from build123d import *

# Parameters (mm, degrees)
SKETCH010_W     = 220
SKETCH010_H     = 102
SKETCH010_W_2   = 150
SKETCH010_H_2   = 6
PAD006_DEPTH    = 10
SKETCH012_W     = 30
SKETCH012_H     = 102
SKETCH012_W_2   = 50
PAD007_DEPTH    = 19.5
CHAMFER001_SIZE = 1
SKETCH_R        = 2.55
HOLE_DEPTH      = 29.501


with BuildPart() as part:
    # Sketch010 → Pad006 (new body)
    with BuildSketch(Plane.XY):
        with BuildLine():
            Line((-150, 71), (-150, -71))
            ThreePointArc((-150, -71), (-148.828427, -73.828427), (-146, -75))
            Line((-146, -75), (146, -75))
            ThreePointArc((146, -75), (148.828427, -73.828427), (150, -71))
            Line((150, -71), (150, 71))
            ThreePointArc((150, 71), (148.828427, 73.828427), (146, 75))
            Line((146, 75), (-146, 75))
            ThreePointArc((-146, 75), (-148.828427, 73.828427), (-150, 71))
        make_face()
        with Locations((10, 0)):
            Rectangle(SKETCH010_W, SKETCH010_H, mode=Mode.SUBTRACT)
        with Locations((-25, 63)):
            Rectangle(SKETCH010_W_2, SKETCH010_H_2, mode=Mode.SUBTRACT)
        with Locations((-25, -63)):
            Rectangle(SKETCH010_W_2, SKETCH010_H_2, mode=Mode.SUBTRACT)
    extrude(amount=PAD006_DEPTH)

    # Sketch012 (on Face21 of Pad006) → Pad007 (join)
    with BuildSketch(Plane(origin=(0, 0, 0), x_dir=(1, 0, 0), z_dir=(0, 0, -1))):
        with Locations((135, 0)):
            Rectangle(SKETCH012_W, SKETCH012_H)
        with Locations((-125, 0)):
            Rectangle(SKETCH012_W_2, SKETCH012_H)
    extrude(amount=PAD007_DEPTH)

    # Chamfer001
    chamfer001_edges = [part.edges().sort_by_distance(p)[0] for p in [
        (-25, -66, 0),
        (-100, -63, 0),
        (-25, -60, 0),
        (50, -63, 0),
        (50, 63, 0),
        (-25, 66, 0),
        (-25, 60, 0),
        (-100, 63, 0),
        (-150, 0, -19.5),
        (-125, 51, -19.5),
        (-100, 0, -19.5),
        (-125, -51, -19.5),
        (120, 0, -19.5),
        (135, 51, -19.5),
        (150, 0, -19.5),
        (135, -51, -19.5),
        (0, -75, 0),
        (0, 75, 0),
        (10, -51, 0),
        (10, 51, 0),
        (-150, 0, 10),
        (-148.828427, -73.828427, 10),
        (0, -75, 10),
        (148.828427, -73.828427, 10),
        (150, 0, 10),
        (148.828427, 73.828427, 10),
        (0, 75, 10),
        (-148.828427, 73.828427, 10),
        (-100, 0, 10),
        (10, -51, 10),
        (120, 0, 10),
        (10, 51, 10),
        (-100, -63, 10),
        (-25, -66, 10),
        (50, -63, 10),
        (-25, -60, 10),
        (-100, 63, 10),
        (-25, 60, 10),
        (50, 63, 10),
        (-25, 66, 10),
    ]]
    chamfer(chamfer001_edges, length=CHAMFER001_SIZE)

    # Sketch (on Face15 of Chamfer001) → Hole (cut, through all)
    with BuildSketch(Plane.XY.offset(10)):
        with Locations((-130, 0)):
            Circle(SKETCH_R)
    extrude(amount=-HOLE_DEPTH, mode=Mode.SUBTRACT)


solid = part.part
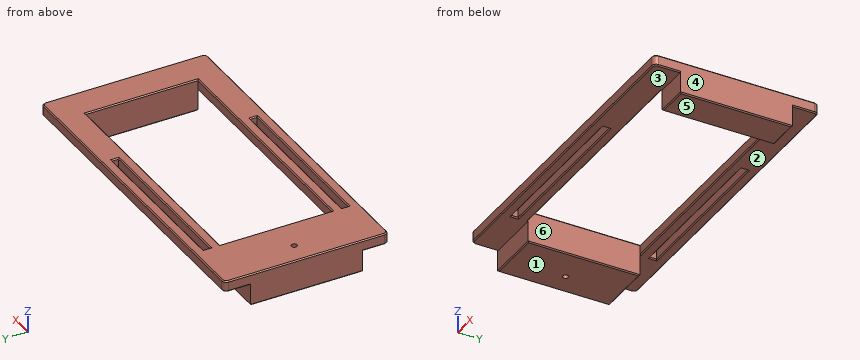
Design review of the part built by this model. Coordinates are the model's own, in mm. Face numbers are marked on the shaded views. A direction names the side the tool comes from. Round coordinates to 2 decimals unless told otherwise and drop trailing zeros. Write each loop counter-clockwise with the first axis right and the second up, starting at its lowest first coordinate (ties: lowest second). Pieces come first, ordered by that corner, then holes. Notation, with made-up numbers: (69, -20) - (91, -20) arc R17 cw to (91, -16) - close; hole circle Ø9 at (63, -20). An arc over 180 degrees is marked (long way). Return JSON: item names as keys, results as strings. Group by question number.
Item 1: Machinability: for the marked faces 1, 2 and 3, which of the approach directions +Z, -Z, +X, -X, +Y, -Y give a long, thin tool a straight path to every point of the face, cutting with its end or side? Answer none if there is none.
Item 2: We need section A-A on y = 31.5. Write out the cut boundary in (x, z).
Item 3: Insertion check: P1, Ø10, axis at x = 113.5, y = -24, coming from the -Z side; P2, Ø3, axis at x = 106, z = 0, coming from the +Y side; P3, Ø15.5, axis at x = -120.5, z = -10, coming from the -Y side; P4, Ø7, axis at x = -50, y = 58.5, coming from the -Z side. Each pin has a flat end and moves straight along its axis. Give the tip position at first contact, or say it passes through.
Item 4: The part is to be moulded in two halves that separate along X. For the marked faces 4, 5 and 6, say which applies: pulls with the +X half, pulls with the -X half, needs draft (parallel to the pull), parting line crosses it, or undercut.
Item 5: We need section B-B on z = -6.5. Write out the cut boundary in (x, y), and give its area (3 significant figures).
Item 6: For probe 1 along Y at (x, z) = (-13.5, 7.75); probe 2 along X at (y, z) = (-24.5, 0); probe 3 along Y at (x, z) = (-130, -4), list the stretches that pass through material, from the lowest coordinate up. Write a range as [from, to].
Item 7: We need section C-C on x = 101. Write out the cut boundary in (y, z).
Model answer:
{
 "1": {"face 1": "-Z, +X, -X, +Y, -Y", "face 2": "-Z, +X, -X, +Y", "face 3": "-Z, +X, -X, -Y"},
 "2": {"outline": "(-150, -18.5) - (-149, -19.5) - (-101, -19.5) - (-100, -18.5) - (-100, 9) - (-101, 10) - (-149, 10) - (-150, 9) - close; (120, -18.5) - (121, -19.5) - (149, -19.5) - (150, -18.5) - (150, 9) - (149, 10) - (121, 10) - (120, 9) - close"},
 "3": {"P1": "passes through", "P2": "stops at y = 75", "P3": "stops at y = -51", "P4": "stops at z = 0"},
 "4": {"face 4": "pulls with the +X half", "face 5": "needs draft", "face 6": "undercut"},
 "5": {"outline": "(-150, -51) - (-100, -51) - (-100, 51) - (-150, 51) - close; (120, -51) - (150, -51) - (150, 51) - (120, 51) - close; hole circle Ø5.1 at (-130, 0)", "area": "8,140 mm²"},
 "6": {"probe 1": "y = [-75, -66], [-60, -51], [51, 60], [66, 75]", "probe 2": "x = [-150, -100], [120, 150]", "probe 3": "y = [-51, -2.55], [2.55, 51]"},
 "7": {"outline": "(-75, 1) - (-74, 0) - (-52, 0) - (-51, 1) - (-51, 9) - (-52, 10) - (-74, 10) - (-75, 9) - close; (51, 1) - (52, 0) - (74, 0) - (75, 1) - (75, 9) - (74, 10) - (52, 10) - (51, 9) - close"}
}
